Design review of the part built by this model. Coordinates are the model's own, in mm. A direction names the side the tool comes from. Coordinates: 2 decimals unless noted, no trailing zeros. Loops run counter-clockwise (first coordinate to the right, second up) from the corner with the lowest first, then second, coordinate; pieces in that order, holes last. Notation, with made-up numbers: (-3.5, 26.25) -> (5.5, 26.25) arc R18 cw to (5.5, 46.25) -> close; hole circle Ø1 at (80.25, 50.5). An arc over 180 degrees is marked (long way). Answer as a JSON object with one key per item and string values.
```python
from build123d import *

# Parameters (mm, degrees)
MODEL_R             = 4
MODEL_W             = 4.999999889
MODEL_H             = 5.349997431
MODEL_H_2           = 5.350001156
BOSS_EXTRUDE1_DEPTH = 5.35


with BuildPart() as part:
    # Model → Boss-Extrude1 (new body)
    with BuildSketch(Plane.XY):
        Polygon((14.000000432, 127.499997616), (14.000000432, 150.00000596), (0, 150.00000596), (0, 0), (14.000000432, 0), (14.000000432, 22.500000894), (19.349999726, 22.500000894), (19.349999726, 42.500000447), (14.000000432, 42.500000447), (14.000000432, 64.999997616), (19.349999726, 64.999997616), (19.349999726, 85.000000894), (14.000000432, 85.000000894), (14.000000432, 107.500001788), (19.349999726, 107.500001788), (19.349999726, 127.499997616), align=None)
        with Locations((7, 11.5)):
            Circle(MODEL_R, mode=Mode.SUBTRACT)
        with Locations((7, 138.5)):
            Circle(MODEL_R, mode=Mode.SUBTRACT)
        with Locations((6.999999751, 54.250000044)):
            Rectangle(MODEL_W, MODEL_H, mode=Mode.SUBTRACT)
        with Locations((6.999999751, 95.750000328)):
            Rectangle(MODEL_W, MODEL_H_2, mode=Mode.SUBTRACT)
        Polygon((1.500000013, 71.82457298), (7.000000216, 68.649150431), (12.500000186, 71.82457298), (12.500000186, 78.175425529), (7.000000216, 81.350855529), (1.500000013, 78.175425529), align=None, mode=Mode.SUBTRACT)
    extrude(amount=BOSS_EXTRUDE1_DEPTH)


solid = part.part
```
1) Add section C-C, the plane y = 45. Give the boundary of the cut face in (x, z), and give its area (3 significant figures).
Completed:
{"outline": "(0, 0) -> (14, 0) -> (14, 5.35) -> (0, 5.35) -> close", "area": "74.9 mm²"}
2) Wall thickness on probe 1 along Y at (x, z) = (15, 4.7); probe 2 along X at (y, z) = (55.5, 4); probe 3 along Y at (x, z) = (5.75, 1.4) (3 decimals): over which ranges is each line inside the solid? List them lowest first.
Completed:
{"probe 1": "22.5 to 42.5, 65 to 85, 107.5 to 127.5", "probe 2": "0 to 4.5, 9.5 to 14", "probe 3": "0 to 7.7, 15.3 to 51.575, 56.925 to 69.371, 80.629 to 93.075, 98.425 to 134.7, 142.3 to 150"}
3) For faces 1 (the flat face through (14, 139, 3)), 2 (the flat face through (9.5, 54, 3)), 3 (the flat face through (17, 85, 3)), list the 3-axis set-ups (+Z, -Z, +X, -X, +Y, -Y) from which the entire face can be reached by the end or side of a thin tool; tool diameter is ignored.
Completed:
{"face 1": "+Z, -Z, +X, +Y", "face 2": "+Z, -Z", "face 3": "+Z, -Z, +X"}
4) Add section B-B, the plane z = 4. Count the separate pieces of the cut face and the enclosed holes in it, and give its area (3 significant figures).
Completed:
{"separate pieces": "1", "enclosed holes": "5", "area": "2,160 mm²"}
5) Clearance check with flat-ended pins moving along their axes: pin 1 Ø3 at (y, z) = (134, 4) entering from -X; pin 2 Ø2 at (y, z) = (89.5, 4.5) entering from +X; pin 3 Ø1.5 at (x, z) = (16, 4) entering from +Y; pin 4 Ø2.5 at (x, z) = (17.5, 3) entering from -Y. State where each tip first meets the part, or that it passes through.
Completed:
{"pin 1": "x = 0", "pin 2": "x = 14", "pin 3": "y = 127.5", "pin 4": "y = 22.5"}
6) The part is to be moulded in two halves that separate along X. For faces 4 (the flat face through (17, 22.5, 3)), 5 (the flat face through (14, 11, 3)), 6 (the flat face through (1.5, 75, 3)), say which applies: pulls with the +X half, pulls with the -X half, needs draft (parallel to the pull), parting line crosses it, or undercut.
Completed:
{"face 4": "needs draft", "face 5": "pulls with the +X half", "face 6": "undercut"}
7) Add section A-A, the plane y = 11.5. Give the boundary of the cut face in (x, z).
Completed:
{"outline": "(0, 0) -> (3, 0) -> (3, 5.35) -> (0, 5.35) -> close; (11, 0) -> (14, 0) -> (14, 5.35) -> (11, 5.35) -> close"}
